```python
from build123d import *

# Parameters (mm, degrees)
BOSS_EXTRUDE1_DEPTH  = 4.75
M2_CLEARANCE_HOLE1_D = 2.4
CUT_EXTRUDE1_DEPTH   = 1.2
SKETCH5_W            = 10
SKETCH5_H            = 15
BOSS_EXTRUDE2_DEPTH  = 2
CUT_EXTRUDE2_DEPTH   = 2
FILLET1_R            = 3
FILLET2_R            = 0.5


with BuildPart() as part:
    # Sketch1 → Boss-Extrude1 (new, symmetric)
    with BuildSketch(Plane.XY):
        Polygon((-16.53737418, 17.07), (-16.53737418, 27.07), (-15.53737418, 27.07), (-15.53737418, 29.07), (-19.53737418, 29.07), (-19.53737418, 0), (-19.53737418, -8.11), (-11.42737418, -8.11), (0.46262582, -8.11), (0.46262582, -6.11), (-15.42737418, -6.11), (-15.53737418, -6.11), (-15.53737418, 14.07), (-15.53737418, 17.07), align=None)
    extrude(amount=BOSS_EXTRUDE1_DEPTH, both=True)

    # M2 Clearance Hole1 (through all)
    with Locations(Plane(origin=(-16.53737418, 22.07, 2.5), x_dir=(0, 1, 0), z_dir=(1, 0, 0))):
        with Locations((0, 0), (0, -5)):
            Hole(M2_CLEARANCE_HOLE1_D / 2)

    # Sketch4 → Cut-Extrude1 (cut)
    with BuildSketch(Plane(origin=(-16.53737418, 0, 0), x_dir=(0, 0, -1), z_dir=(1, 0, 0))):
        with BuildLine():
            Line((-2.5, 24.07), (-4.75, 24.07))
            Line((-4.75, 24.07), (-4.75, 20.07))
            Line((-4.75, 20.07), (-2.5, 20.07))
            ThreePointArc((-2.5, 20.07), (-0.5, 22.07), (-2.5, 24.07))
        make_face()
        with BuildLine():
            Line((4.75, 20.07), (2.5, 20.07))
            ThreePointArc((2.5, 20.07), (0.5, 22.07), (2.5, 24.07))
            Line((2.5, 24.07), (4.75, 24.07))
            Line((4.75, 24.07), (4.75, 20.07))
        make_face()
    extrude(amount=-CUT_EXTRUDE1_DEPTH, mode=Mode.SUBTRACT)

    # Sketch5 → Boss-Extrude2 (add)
    with BuildSketch(Plane.XZ.offset(8.11)):
        with Locations((-4.53737418, 0)):
            Rectangle(SKETCH5_W, SKETCH5_H)
    extrude(amount=-BOSS_EXTRUDE2_DEPTH)

    # Sketch6 → Cut-Extrude2 (cut)
    with BuildSketch(Plane(origin=(0, -6.11, 0), x_dir=(1, 0, 0), z_dir=(0, 1, 0))):
        with BuildLine():
            Line((-3.28737418, -5.2), (-5.78737418, -5.2))
            ThreePointArc((-5.78737418, -5.2), (-6.98737418, -4), (-5.78737418, -2.8))
            Line((-5.78737418, -2.8), (-3.28737418, -2.8))
            ThreePointArc((-3.28737418, -2.8), (-2.08737418, -4), (-3.28737418, -5.2))
        make_face()
        with BuildLine():
            Line((-3.28737418, 5.2), (-5.78737418, 5.2))
            ThreePointArc((-5.78737418, 5.2), (-6.98737418, 4), (-5.78737418, 2.8))
            Line((-5.78737418, 2.8), (-3.28737418, 2.8))
            ThreePointArc((-3.28737418, 2.8), (-2.08737418, 4), (-3.28737418, 5.2))
        make_face()
    extrude(amount=-CUT_EXTRUDE2_DEPTH, mode=Mode.SUBTRACT)

    # Fillet1
    fillet1_edges = [part.edges().sort_by_distance(p)[0] for p in [
        (-15.53737418, -6.11, 0),
        (-19.53737418, -8.11, 0),
    ]]
    fillet(fillet1_edges, radius=FILLET1_R)

    # Fillet2
    fillet2_edges = [part.edges().sort_by_distance(p)[0] for p in [
        (-16.53737418, 27.07, 0),
        (-16.53737418, 17.07, 0),
    ]]
    fillet(fillet2_edges, radius=FILLET2_R)


solid = part.part
```
Here's how the part is built. I have some questions about the finished solid (model axes, mm). A direction names the side the tool comes from. Round coordinates to 2 decimals unless told otherwise and drop trailing zeros. Write each loop counter-clockwise with the first axis right and the second up, starting at its lowest first coordinate (ties: lowest second). Pieces come first, ordered by that corner, then holes.
Q1. If we section it at D-D on y = 7.5: Write out the boundary of the cut face in (x, z).
Q2. Will these pins go through, and if not, where does the flat tip stop? P1, Ø1, axis at y = 28.5, z = -2, coming from the +X side; P2, Ø3, axis at x = -16.5, y = 18, coming from the -Z side; P3, Ø4, axis at y = 20.5, z = 4, coming from the +X side; P4, Ø5, axis at x = -12, y = 19, coming from the +Z side.
Q3. If we section it at B-B on y = 22.07: Write out the boundary of the cut face in (x, z), plus the area to 3 significant figures.
Q4. Please list where these lines run through material, in increasing order: probe 1 along Z at (x, y) = (-18.4, 22.07); probe 2 along Z at (x, y) = (-17.5, 25); probe 3 along Y at (x, z) = (-2.75, 6.5).
Q5. If we section it at A-A on x = -4.75: Write out the boundary of the cut face in (y, z).
Q6. Which directions (+Z, -Z, +X, -X, +Y, -Y) give clear straight access to the entire face, cutting with the end or side of a thin tool? Please do faces 5 (the flat face through (-17.737, 23, 4)), 6 (the flat face through (-5, -7, -5.2)), 7 (the flat face through (-17.737, 23, -4)).
Q7. If we section it at C-C on z = 0: Write out the boundary of the cut face in (x, y).
Q8. If we mould it in two halves opening along Y, with no side actions, what happens to faces 1 (the cylindrical face through (-18.64, -7.25, 0.07)), 2 (the flat face through (-5, -7, -7.5)), 3 (the flat face through (-18, 29.07, 0)), 4 (the flat face through (-17, 24.07, 4))? For each: +Y half, -Y half, draft (parallel to the pull), parting line (faces both ways), or undercut.
Answer below:
1. outline: (-19.54, -4.75) - (-15.54, -4.75) - (-15.54, 4.75) - (-19.54, 4.75) - close
2. P1: stops at x = -15.54
2. P2: stops at z = -4.75
2. P3: stops at x = -16.54
2. P4: passes through
3. outline: (-19.54, -4.75) - (-17.74, -4.75) - (-17.74, -3.7) - (-19.54, -3.7) - close; (-19.54, -1.3) - (-17.74, -1.3) - (-17.74, -0.5) - (-16.54, -0.5) - (-16.54, 0.5) - (-17.74, 0.5) - (-17.74, 1.3) - (-19.54, 1.3) - close; (-19.54, 3.7) - (-17.74, 3.7) - (-17.74, 4.75) - (-19.54, 4.75) - close
3. area: 9.66 mm2
4. probe 1: z = -4.75 to -3.7, -1.3 to 1.3, 3.7 to 4.75
4. probe 2: z = -4.75 to 4.75
4. probe 3: y = -8.11 to -6.11
5. outline: (-8.11, -7.5) - (-6.11, -7.5) - (-6.11, -5.2) - (-8.11, -5.2) - close; (-8.11, -2.8) - (-6.11, -2.8) - (-6.11, 2.8) - (-8.11, 2.8) - close; (-8.11, 5.2) - (-6.11, 5.2) - (-6.11, 7.5) - (-8.11, 7.5) - close
6. face 5: +Z, +X
6. face 6: +Y, -Y
6. face 7: -Z, +X
7. outline: (-19.54, -5.11) arc R3 ccw to (-16.54, -8.11) - (0.46, -8.11) - (0.46, -6.11) - (-12.54, -6.11) arc R3 cw to (-15.54, -3.11) - (-15.54, 17.07) - (-16.04, 17.07) arc R0.5 cw to (-16.54, 17.57) - (-16.54, 26.57) arc R0.5 cw to (-16.04, 27.07) - (-15.54, 27.07) - (-15.54, 29.07) - (-19.54, 29.07) - close
8. face 1: -Y half
8. face 2: draft
8. face 3: +Y half
8. face 4: undercut
